```python
from build123d import *

# Parameters (mm, degrees)
BOSS_EXTRUDE1_START = -0.9
SKETCH2_W           = 0.3
SKETCH2_H           = 0.56
BOSS_EXTRUDE1_DEPTH = 4
BOSS_EXTRUDE2_DEPTH = 4.5
SKETCH4_W           = 0.4
SKETCH4_H           = 0.24
BOSS_EXTRUDE3_DEPTH = 2.5


with BuildPart() as part:
    # Sketch2 → Boss-Extrude1 (new body)
    with BuildSketch(Plane.XY.offset(BOSS_EXTRUDE1_START)):
        with BuildLine():
            Line((2.3, 2.75), (-2.3, 2.75))
            Line((-2.3, 2.75), (-2.3, 1.85))
            ThreePointArc((-2.3, 1.85), (-2.080330086, 1.319669914), (-1.55, 1.1))
            Line((-1.55, 1.1), (1.55, 1.1))
            ThreePointArc((1.55, 1.1), (2.080330086, 1.319669914), (2.3, 1.85))
            Line((2.3, 1.85), (2.3, 2.75))
        make_face()
        with Locations((-1.65, 1.92)):
            Rectangle(SKETCH2_W, SKETCH2_H, mode=Mode.SUBTRACT)
        with Locations((-0.83, 1.92)):
            Rectangle(SKETCH2_W, SKETCH2_H, mode=Mode.SUBTRACT)
        with Locations((0, 1.92)):
            Rectangle(SKETCH2_W, SKETCH2_H, mode=Mode.SUBTRACT)
        with Locations((0.83, 1.92)):
            Rectangle(SKETCH2_W, SKETCH2_H, mode=Mode.SUBTRACT)
        with Locations((1.65, 1.92)):
            Rectangle(SKETCH2_W, SKETCH2_H, mode=Mode.SUBTRACT)
    extrude(amount=-BOSS_EXTRUDE1_DEPTH)

    # Sketch3 → Boss-Extrude2 (add)
    with BuildSketch(Plane(origin=(0, 0, -4.9), x_dir=(-1, 0, 0), z_dir=(0, 0, -1))):
        with BuildLine():
            Line((-3.3, 3.7), (3.3, 3.7))
            ThreePointArc((3.3, 3.7), (3.476776695, 3.626776695), (3.55, 3.45))
            Line((3.55, 3.45), (3.55, 0))
            Line((3.55, 0), (-3.55, 0))
            Line((-3.55, 0), (-3.55, 3.45))
            ThreePointArc((-3.55, 3.45), (-3.476776695, 3.626776695), (-3.3, 3.7))
        make_face()
    extrude(amount=BOSS_EXTRUDE2_DEPTH)

    # Sketch4 → Boss-Extrude3 (add)
    with BuildSketch(Plane(origin=(0, 0, -9.4), x_dir=(-1, 0, 0), z_dir=(0, 0, -1))):
        with Locations((-0.77, 3.11)):
            Rectangle(SKETCH4_W, SKETCH4_H)
        with Locations((0.77, 3.11)):
            Rectangle(SKETCH4_W, SKETCH4_H)
        with Locations((0, 1.42)):
            Rectangle(SKETCH4_W, SKETCH4_H)
        with Locations((1.73, 1.42)):
            Rectangle(SKETCH4_W, SKETCH4_H)
        with Locations((-1.73, 1.42)):
            Rectangle(SKETCH4_W, SKETCH4_H)
    extrude(amount=BOSS_EXTRUDE3_DEPTH)


solid = part.part
```
Check sheet for the modelled part. Datum: model origin and axes. Units: mm. A direction names the side the tool comes from. Round coordinates to 2 decimals unless told otherwise and drop trailing zeros. Order: outer loops, then holes, each group sorted by start corner. A loop starts at its lowest first (then second) coordinate and runs counter-clockwise, first axis right, second up. Notation, with made-up numbers: (37.5, -19.5) - (82.5, -19.5) arc R26 cw to (82.5, 6.5) - close; hole circle Ø3 at (2.5, 80). An arc over 180 degrees is marked (long way). Answer as CSV lines item,"result". Start each with the question number.
1) Depth check by flat-ended pin: pin 1 (1.5 mm diameter, centred on x = -0.5, y = 3, fed in from -Z); pin 2 (0.6 mm diameter, centred on y = 2, z = -3, fed in from -X). Enter the tip coordinate at first touch or a pass-through.
2) Section check B-B (z = -10.5). Record the cut outline in (x, y).
3) Section check D-D (y = 0.5). Record the cut outline in (x, z), then the cut area to 4 significant figures.
4) Section check C-C (x = 1.25). Record the cut outline in (y, z), then the cut area to 4 significant figures.
5) Scan lines: probe 1 along Z at (x, y) = (0, 2.95); probe 2 along Z at (x, y) = (2, 2.45); probe 3 along X at (y, z) = (2.65, -4.5). Record each from-to range of solid material in increasing order.
6) Section check A-A (z = -4.5). Record the cut outline in (x, y), then the cut area to 3 significant figures.
7) Tool access check on faces 1 (the face through (0, 2.75, -3)), 2 (the face through (0, 1.1, -3)), 3 (the face through (-2.3, 2.3, -2.9)). Record the directions out of +Z, -Z, +X, -X, +Y, -Y that give a thin tool (end or side, any length) a straight path to the whole face; none if there is none.
Determined:
1,pin 1,"z = -11.9"
1,pin 2,"x = -2.3"
2,outline,"(-1.93, 1.3) - (-1.53, 1.3) - (-1.53, 1.54) - (-1.93, 1.54) - close; (-0.97, 2.99) - (-0.57, 2.99) - (-0.57, 3.23) - (-0.97, 3.23) - close; (-0.2, 1.3) - (0.2, 1.3) - (0.2, 1.54) - (-0.2, 1.54) - close; (0.57, 2.99) - (0.97, 2.99) - (0.97, 3.23) - (0.57, 3.23) - close; (1.53, 1.3) - (1.93, 1.3) - (1.93, 1.54) - (1.53, 1.54) - close"
3,outline,"(-3.55, -9.4) - (3.55, -9.4) - (3.55, -4.9) - (-3.55, -4.9) - close"
3,area,"31.95 mm^2"
4,outline,"(0, -9.4) - (3.7, -9.4) - (3.7, -4.9) - (2.75, -4.9) - (2.75, -0.9) - (1.1, -0.9) - (1.1, -4.9) - (0, -4.9) - close"
4,area,"23.25 mm^2"
5,probe 1,"-9.4 to -4.9"
5,probe 2,"-9.4 to -0.9"
5,probe 3,"-2.3 to 2.3"
6,outline,"(-2.3, 1.85) arc R0.75 ccw to (-1.55, 1.1) - (1.55, 1.1) arc R0.75 ccw to (2.3, 1.85) - (2.3, 2.75) - (-2.3, 2.75) - close; hole (-1.8, 1.64) - (-1.5, 1.64) - (-1.5, 2.2) - (-1.8, 2.2) - close; hole (-0.98, 1.64) - (-0.68, 1.64) - (-0.68, 2.2) - (-0.98, 2.2) - close; hole (-0.15, 1.64) - (0.15, 1.64) - (0.15, 2.2) - (-0.15, 2.2) - close; hole (0.68, 1.64) - (0.98, 1.64) - (0.98, 2.2) - (0.68, 2.2) - close; hole (1.5, 1.64) - (1.8, 1.64) - (1.8, 2.2) - (1.5, 2.2) - close"
6,area,"6.51 mm^2"
7,face 1,"+Z, +X, -X, +Y"
7,face 2,"+Z, +X, -X, -Y"
7,face 3,"+Z, -X, +Y, -Y"
